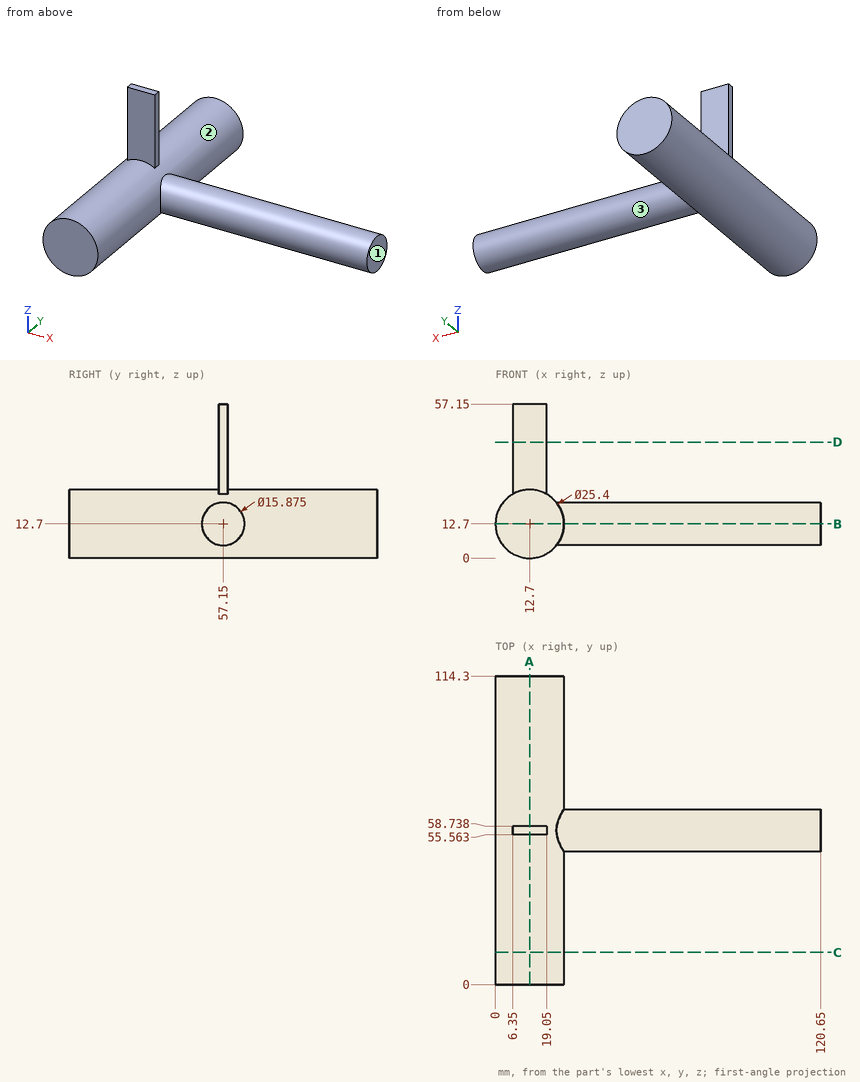
The figure shows three views and two pictorial views of one solid part (mm, origin at its lowest corner). Answer the questions. A direction names the side the tool comes from. Give positions to 0.01 mm unless a question says otherwise; leave off trailing zeros. Loops run counter-clockwise (first coordinate to the right, second up) from the corner with the lowest first, then second, coordinate; pieces in that order, holes last. Notation, with made-up numbers: (40, 37.5) -> (96, 37.5) arc R35 ccw to (96, 73.5) -> close; hole circle Ø5 at (25.25, 75). An arc over 180 degrees is marked (long way). Put each result on its own line as item: value. Start each with the question number.
Item 1: The part is cut by section C-C (y = 12). Give the vertices of the cut face in (x, z).
Item 2: The part is cut by section B-B (z = 12.7). Give the vertices of the cut face in (x, y).
Item 3: Which of the six approach directions +Z, -Z, +X, -X, +Y, -Y give full straight-line access (tool end or side, diameter ignored) to the marked faces 1, 2 and 3?
Item 4: The part is cut by section A-A (x = 12.7). Give the vertices of the cut face in (y, z), then the cut area to 3 significant figures.
Item 5: Each of these flat-tipped pins is pushed along its axis until it touches: P1, Ø3.5, axis at y = 57.5, z = 46, coming from the +X side; P2, Ø1, axis at y = 66, z = 13, coming from the +X side; P3, Ø6, axis at y = 48, z = 25, coming from the +X side. Where does it stop, or does it pass through?
Item 6: The part is cut by section D-D (z = 43). Give the vertices of the cut face in (x, y).
Item 7: Find the intervals of material crossed by L1, parallel to Y at x = 48, z = 13; L2, parallel to X at y = 61.5, z = 13; L3, parallel to X at y = 69, z = 6.5 (1 decimal), in increasing order. Write a range as [from, to].
Answers below:
1. outline: circle Ø25.4 at (12.7, 12.7)
2. outline: (0, 0) -> (25.4, 0) -> (25.4, 49.21) -> (120.65, 49.21) -> (120.65, 65.09) -> (25.4, 65.09) -> (25.4, 114.3) -> (0, 114.3) -> close
3. face 1: +Z, -Z, +X, +Y, -Y
3. face 2: none
3. face 3: +X
4. outline: (0, 0) -> (114.3, 0) -> (114.3, 25.4) -> (58.74, 25.4) -> (58.74, 57.15) -> (55.56, 57.15) -> (55.56, 25.4) -> (0, 25.4) -> close
4. area: 3,000 mm2
5. P1: x = 19.05
5. P2: x = 25.4
5. P3: x = 21.35
6. outline: (6.35, 55.56) -> (19.05, 55.56) -> (19.05, 58.74) -> (6.35, 58.74) -> close
7. L1: [49.22, 65.08]
7. L2: [0, 120.65]
7. L3: [1.6, 23.8]
